Verification items for the finished model (mm, model axes). A direction names the side the tool comes from. Coordinates: 2 decimals unless noted, no trailing zeros. Order: outer loops, then holes, each group sorted by start corner. A loop starts at its lowest first (then second) coordinate and runs counter-clockwise, first axis right, second up. Notation, with made-up numbers: (-30.5, 52.25) -> (-8.5, 52.25) arc R14 cw to (-8.5, 77.25) -> close; hole circle Ø8 at (84.5, 52). An arc over 180 degrees is marked (long way). Write item = value, one per line. Start each with the question number.
1. Cross-section at A-A on x = -30.5. Record the cut outline in (y, z), plus the area to 3 significant figures.
2. Cross-section at B-B on y = 64. Give the number of separate pieces and of enclosed holes in the cut face, plus the area to 3 significant figures.
3. Thickness scan on line 1 along X through (y, z) = (66, 27); line 2 along Y through (x, z) = (-39, -11); line 3 along Y through (x, z) = (-35, -20). Record the ranges inside material, lowest first. Write a range as from..to.
4. Cross-section at C-C on x = -57.5. Record the cut outline in (y, z), plus the area to 3 significant figures.
5. Set-up check for faces 4 (the flat face through (-44, 36, -18.333)), 5 (the flat face through (-57, 66.5, -20)), 6 (the cylindrical face through (-46.677, 73.768, 47.572)), 7 (the cylindrical face through (-21.5, 12.6, 50.1)): record each of +Z, -Z, +X, -X, +Y, -Y from which the full face is reachable in a straight line by a thin tool's end or side.
6. Go/stop test with flat-tipped pins: P1, Ø3, axis at x = -61.95, y = 64, coming from the -Z side; P2, Ø4, axis at x = -54.5, y = 69, coming from the +Z side; P3, Ø12, axis at x = -39, z = -8, coming from the -Y side. Record where each tip stops, or that it passes through.
7. Release check for a two-part mould opening along Z. For faces 1 (the cylindrical face through (-22.39, 36.76, -17.76)), 2 (the flat face through (-19.29, 38, 18)), 3 (the cylindrical face through (-21.54, 64.78, 50.65)) record: +Z half, -Z half, draft (parallel to the pull), parting line (faces both ways), or undercut.
from build123d import *

# Parameters (mm, degrees)
BOSS_EXTRUDE1_DEPTH = 75
FILLET1_R           = 2
SKETCH4_R           = 1.15
CUT_EXTRUDE2_DEPTH  = 5
BOSS_EXTRUDE2_DEPTH = 58
SKETCH7_W           = 12
SKETCH7_H           = 80
CUT_EXTRUDE3_DEPTH  = 5
SKETCH8_W           = 2.5
SKETCH8_H           = 75
BOSS_EXTRUDE3_DEPTH = 20
SKETCH10_W          = 71.647703853
SKETCH10_H          = 2.5
BOSS_EXTRUDE4_DEPTH = 20
SKETCH12_W          = 3.098039447
SKETCH12_H          = 2.1077236
CUT_EXTRUDE4_DEPTH  = 58
SKETCH13_W          = 11.16
SKETCH13_H          = 75
BOSS_EXTRUDE6_DEPTH = 2
SKETCH14_R          = 1
SKETCH14_R_2        = 0.99762978
CUT_EXTRUDE5_DEPTH  = 10
CHAMFER2_SIZE       = 1
SKETCH16_W          = 2.5
SKETCH16_H          = 75
BOSS_EXTRUDE7_DEPTH = 10
SKETCH17_W          = 71.3
SKETCH17_H          = 2.5
BOSS_EXTRUDE8_DEPTH = 10
SKETCH18_R          = 1.15
CUT_EXTRUDE7_DEPTH  = 4
CUT_EXTRUDE8_DEPTH  = 10
BOSS_EXTRUDE9_START = 2.5
SKETCH21_W          = 18.75
SKETCH21_H          = 75
SKETCH21_R          = 1.15
BOSS_EXTRUDE9_DEPTH = 2.5
CUT_EXTRUDE10_DEPTH = 2.5
CHAMFER3_SIZE       = 1
FILLET2_START       = -1
FILLET2_DEPTH       = 77


with BuildPart() as part:
    # Sketch1 → Boss-Extrude1 (new body)
    with BuildSketch(Plane(origin=(0, 0, 0), x_dir=(1, 0, 0), z_dir=(0, 1, 0))):
        with BuildLine():
            Line((-23.765673143, -52.966666667), (-21.11640892, -52.966666667))
            ThreePointArc((-21.11640892, -52.966666667), (-19.749251579, -47.460938782), (-19.289506454, -41.806666667))
            Line((-19.289506454, -41.806666667), (-19.289506454, 18.333333333))
            Line((-19.289506454, 18.333333333), (-19.289506454, 20.833333333))
            Line((-19.289506454, 20.833333333), (-34.949506454, 20.833333333))
            Line((-34.949506454, 20.833333333), (-34.949506454, 18.333333333))
            Line((-34.949506454, 18.333333333), (-21.789506454, 18.333333333))
            Line((-21.789506454, 18.333333333), (-21.789506454, -41.806666667))
            ThreePointArc((-21.789506454, -41.806666667), (-22.287361349, -47.473474295), (-23.765673143, -52.966666667))
        make_face()
    extrude(amount=BOSS_EXTRUDE1_DEPTH)

    # Fillet1
    fillet1_edges = [part.edges().sort_by_distance(p)[0] for p in [
        (-21.789506454, 37.5, -18.333333333),
        (-19.289506454, 37.5, -20.833333333),
    ]]
    fillet(fillet1_edges, radius=FILLET1_R)

    # Sketch4 → Cut-Extrude2 (cut)
    with BuildSketch(Plane(origin=(-19.289506454, 0, 0), x_dir=(0, 0, -1), z_dir=(1, 0, 0))):
        with Locations((-49.806666667, 64)):
            Circle(SKETCH4_R)
        with Locations((-48.955669454, 12.5)):
            Circle(SKETCH4_R)
    extrude(amount=-CUT_EXTRUDE2_DEPTH, mode=Mode.SUBTRACT)

    # Sketch6 → Boss-Extrude2 (add)
    with BuildSketch(Plane(origin=(0, 0, -16.333333333), x_dir=(-1, 0, 0), z_dir=(0, 0, -1))):
        Polygon((19.539506454, 75), (21.539506454, 75), (20.48442105, 77), align=None)
        Polygon((21.539506454, 0), (19.539506454, 0), (20.539506454, -2), align=None)
    extrude(amount=-BOSS_EXTRUDE2_DEPTH)

    # Sketch7 → Cut-Extrude3 (cut)
    with BuildSketch(Plane.ZY.offset(21.789506454)):
        with Locations((47.806666667, 35)):
            Rectangle(SKETCH7_W, SKETCH7_H)
    extrude(amount=CUT_EXTRUDE3_DEPTH, mode=Mode.SUBTRACT)

    # Sketch8 → Boss-Extrude3 (add)
    with BuildSketch(Plane.ZY.offset(34.949506454)):
        with Locations((-19.583333333, 37.5)):
            Rectangle(SKETCH8_W, SKETCH8_H)
    extrude(amount=BOSS_EXTRUDE3_DEPTH)

    # Sketch10 → Boss-Extrude4 (add)
    with BuildSketch(Plane.ZY.offset(21.789506454)):
        with Locations((17.142814741, 73.75)):
            Rectangle(SKETCH10_W, SKETCH10_H)
    extrude(amount=BOSS_EXTRUDE4_DEPTH)

    # Sketch12 → Cut-Extrude4 (cut)
    with BuildSketch(Plane(origin=(0, 0, -16.333333333), x_dir=(-1, 0, 0), z_dir=(0, 0, -1))):
        with Locations((20.374958132, 76.0538618)):
            Rectangle(SKETCH12_W, SKETCH12_H)
    extrude(amount=-CUT_EXTRUDE4_DEPTH, mode=Mode.SUBTRACT)

    # Sketch13 → Boss-Extrude6 (add)
    with BuildSketch(Plane(origin=(-19.289506454, 0, 0), x_dir=(0, 0, -1), z_dir=(1, 0, 0))):
        with Locations((-47.386666667, 37.5)):
            Rectangle(SKETCH13_W, SKETCH13_H)
    extrude(amount=-BOSS_EXTRUDE6_DEPTH)

    # Sketch14 → Cut-Extrude5 (cut)
    with BuildSketch(Plane.ZY.offset(21.289506454)):
        with Locations((49.806666667, 64)):
            Circle(SKETCH14_R)
        with Locations((48.955669454, 12.5)):
            Circle(SKETCH14_R_2)
    extrude(amount=-CUT_EXTRUDE5_DEPTH, mode=Mode.SUBTRACT)

    # Chamfer2
    chamfer2_edges = [part.edges().sort_by_distance(p)[0] for p in [
        (-19.289506454, 64, 48.806666667),
        (-19.289506454, 12.5, 47.958039674),
    ]]
    chamfer(chamfer2_edges, length=CHAMFER2_SIZE)

    # Sketch16 → Boss-Extrude7 (add)
    with BuildSketch(Plane.ZY.offset(54.949506454)):
        with Locations((-19.583333333, 37.5)):
            Rectangle(SKETCH16_W, SKETCH16_H)
    extrude(amount=BOSS_EXTRUDE7_DEPTH)

    # Sketch17 → Boss-Extrude8 (add)
    with BuildSketch(Plane.ZY.offset(41.789506454)):
        with Locations((17.316666667, 73.75)):
            Rectangle(SKETCH17_W, SKETCH17_H)
    extrude(amount=BOSS_EXTRUDE8_DEPTH)

    # Sketch18 → Cut-Extrude7 (cut)
    with BuildSketch(Plane(origin=(0, 0, -20.833333333), x_dir=(-1, 0, 0), z_dir=(0, 0, -1))):
        with Locations((61.949506454, 64)):
            Circle(SKETCH18_R)
        with Locations((61.949506454, 37.5)):
            Circle(SKETCH18_R)
        with Locations((61.949506454, 11)):
            Circle(SKETCH18_R)
    extrude(amount=-CUT_EXTRUDE7_DEPTH, mode=Mode.SUBTRACT)

    # Sketch20 → Cut-Extrude8 (cut)
    with BuildSketch(Plane(origin=(0, 75, 0), x_dir=(1, 0, 0), z_dir=(0, 1, 0))):
        with BuildLine():
            Line((-46.299506454, -41.906666667), (-49.199506454, -41.906666667))
            Line((-49.199506454, -41.906666667), (-49.199506454, 18.333333333))
            Line((-49.199506454, 18.333333333), (-51.789506454, 18.333333333))
            Line((-51.789506454, 18.333333333), (-51.789506454, -52.966666667))
            Line((-51.789506454, -52.966666667), (-47.849506454, -52.966666667))
            ThreePointArc((-47.849506454, -52.966666667), (-46.665976454, -47.493919967), (-46.299506454, -41.906666667))
        make_face()
    extrude(amount=-CUT_EXTRUDE8_DEPTH, mode=Mode.SUBTRACT)

    # Sketch21 → Boss-Extrude9 (add)
    with BuildSketch(Plane(origin=(0, 0, -20.833333333), x_dir=(-1, 0, 0), z_dir=(0, 0, -1)).offset(BOSS_EXTRUDE9_START)):
        with Locations((55.574506454, 37.5)):
            Rectangle(SKETCH21_W, SKETCH21_H)
        with Locations((61.949506454, 11)):
            Circle(SKETCH21_R, mode=Mode.SUBTRACT)
        with Locations((61.949506454, 37.5)):
            Circle(SKETCH21_R, mode=Mode.SUBTRACT)
        with Locations((61.949506454, 64)):
            Circle(SKETCH21_R, mode=Mode.SUBTRACT)
    extrude(amount=-BOSS_EXTRUDE9_DEPTH)

    # Sketch22 → Cut-Extrude10 (cut)
    with BuildSketch(Plane.XY.offset(-18.333333333)):
        Polygon((-49.199506454, 66.5), (-49.199506454, 72.5), (-49.199506454, 75), (-64.949506454, 75), (-64.949506454, 66.5), align=None)
    extrude(amount=-CUT_EXTRUDE10_DEPTH, mode=Mode.SUBTRACT)

    # Chamfer3
    chamfer3_edges = [part.edges().sort_by_distance(p)[0] for p in [
        (-60.799506454, 37.5, -23.333333333),
        (-60.799506454, 11, -23.333333333),
        (-60.799506454, 64, -23.333333333),
    ]]
    chamfer(chamfer3_edges, length=CHAMFER3_SIZE)

    # Fillet2: read off the stored shape, not the designer's step
    # Fillet2 outline → Fillet2 (cut)
    with BuildSketch(Plane(origin=(0, 0, 0), x_dir=(1, 0, 0), z_dir=(0, 1, 0)).offset(FILLET2_START)):
        with BuildLine():
            add(Edge.make_bspline(
                [(-46.199506454, 20.833333333), (-46.968828273, 23.333333333), (-54.323544859, 23.333333333)],
                knots=[0, 0, 0, 1, 1, 1], degree=2, weights=[1, 0.804399667, 1]))
            Line((-46.199506454, 20.833333333), (-46.199506454, 23.333333333))
            Line((-46.199506454, 23.333333333), (-54.323544859, 23.333333333))
        make_face()
    extrude(amount=FILLET2_DEPTH, mode=Mode.SUBTRACT)


solid = part.part
Worked out:
q1.outline = (0, -20.83) -> (75, -20.83) -> (75, 52.97) -> (72.5, 52.97) -> (72.5, -18.33) -> (0, -18.33) -> close
q1.area = 366 mm²
q2.separate_pieces = 3
q2.enclosed_holes = 0
q2.area = 316 mm²
q3.line_1 = -21.79..-19.29
q3.line_2 = 72.5..75
q3.line_3 = 0..75
q4.outline = (0, -23.33) -> (75, -23.33) -> (75, -20.83) -> (66.5, -20.83) -> (66.5, -18.33) -> (0, -18.33) -> close
q4.area = 354 mm²
q5.face_4 = +Z, -X, -Y
q5.face_5 = +Z, -X, +Y
q5.face_6 = -X, +Y, -Y
q5.face_7 = -X
q6.P1 = -22.68
q6.P2 = -20.83
q6.P3 = 72.5
q7.face_1 = +Z half
q7.face_2 = draft
q7.face_3 = undercut
